from build123d import *

# Parameters (mm, degrees)
BOSS_EXTRUDE1_DEPTH = 3.175
SKETCH3_R           = 2.1
CUT_EXTRUDE1_DEPTH  = 4.175


with BuildPart() as part:
    # Sketch1 → Boss-Extrude1 (new body)
    with BuildSketch(Plane(origin=(0, 0, 0), x_dir=(0, 0, -1), z_dir=(1, 0, 0))):
        with BuildLine():
            Line((-62.23, -8.4201), (62.23, -8.4201))
            Line((62.23, -8.4201), (62.23, 8.4201))
            Line((62.23, 8.4201), (-51.7525, 8.4201))
            ThreePointArc((-51.7525, 8.4201), (-54.8212887, 1.0113887), (-62.23, -2.0574))
            Line((-62.23, -2.0574), (-62.23, -8.4201))
        make_face()
    extrude(amount=BOSS_EXTRUDE1_DEPTH)

    # Sketch3 → Cut-Extrude1 (cut, through all)
    with BuildSketch(Plane.ZY):
        with Locations((-43.18, 2.0701)):
            Circle(SKETCH3_R)
        with Locations((-19.05, 2.0701)):
            Circle(SKETCH3_R)
        with Locations((5.08, 2.0701)):
            Circle(SKETCH3_R)
        with Locations((29.21, 2.0701)):
            Circle(SKETCH3_R)
    extrude(amount=-CUT_EXTRUDE1_DEPTH, mode=Mode.SUBTRACT)


solid = part.part
Could you check a few things on this model? Use its own coordinates, in mm. Give positions to 0.01 mm unless a question says otherwise; leave off trailing zeros. Order: outer loops, then holes, each group sorted by start corner. A loop starts at its lowest first (then second) coordinate and runs counter-clockwise, first axis right, second up. Notation, with made-up numbers: (54, 41) - (67, 41) arc R15 cw to (67, 64) - close; hole circle Ø6 at (61, 73). An arc over 180 degrees is marked (long way). One line per question, with ' | ' between items. Start each with the question number.
Item 1: I want a section at A-A on z = 5.08. Write out the boundary of the cut face in (x, y) (3 decimals).
Item 2: Thinking about a two-plate mould opening in Z: for faces 1 (the flat face through (2, 0, -62.23)), 2 (the cylindrical face through (1.565, 0.792, 27.544)), 3 (the cylindrical face through (1.565, 1.093, 54.74)), which applies, pulls with the +Z half, pulls with the -Z half, needs draft (parallel to the pull), parting line crosses it, or undercut?
Item 3: I'm going to push flat-ended pins straight in: pin 1 Ø3.5 at (y, z) = (2.07, -43.18) entering from +X; pin 2 Ø5.5 at (y, z) = (2.07, -19.05) entering from +X (3 decimals). Where does each tip first touch, or does it pass through?
Item 4: I need wall thicknesses on probe 1 along Z at (x, y) = (1.7, 2.5); probe 2 along Z at (x, y) = (1.15, 1.25); probe 3 along Y at (x, z) = (0.9, -17.5). Which ranges of each line are inside material? Lowest first, please. Write a range as [from, to].
Item 5: I want a section at B-B on x = 2.2. Give the number of separate pieces and of enclosed holes in the cut face, then the cut area to 3 significant figures.
Verdict:
1) outline: (0, -8.42) - (3.175, -8.42) - (3.175, -0.03) - (0, -0.03) - close; (0, 4.17) - (3.175, 4.17) - (3.175, 8.42) - (0, 8.42) - close
2) face 1: pulls with the -Z half | face 2: undercut | face 3: pulls with the +Z half
3) pin 1: through | pin 2: x = 3.175
4) probe 1: [-62.23, -45.24], [-41.12, -21.11], [-16.99, 3.02], [7.14, 27.15], [31.27, 53.59] | probe 2: [-62.23, -45.11], [-41.25, -20.98], [-17.12, 3.15], [7.01, 27.28], [31.14, 54.59] | probe 3: [-8.42, 0.65], [3.49, 8.42]
5) separate pieces: 1 | enclosed holes: 4 | area: 1,950 mm^2
